Autodesk Inventor part; units mm, degrees
ref_plane "YZ Plane" through (0, 0, 0) normal (1, 0, 0) x (0, 1, 0)
ref_plane "XZ Plane" through (0, 0, 0) normal (0, 1, 0) x (-1, 0, 0)
ref_plane "XY Plane" through (0, 0, 0) normal (0, 0, 1) x (1, 0, 0)
sketch "Sketch1" plane through (0, 0, 0) normal (0, 1, 0) x (-1, 0, 0)
  line L0 (14.0131, 53.7275) -> (-24.0869, 53.7275)
  line L1 (-24.0869, 53.7275) -> (-24.0869, -136.7725)
  line L2 (-24.0869, -136.7725) -> (14.0131, -136.7725)
  line L3 (14.0131, -136.7725) -> (14.0131, 53.7275)
  line L4 (-5.0369, 53.7275) -> (-5.0369, -136.7725)
  point P0 (0, 0)
  dimension "d0" = 38.1
  dimension "d1" = 190.5
revolve "Revolution1" add sketch "Sketch1" angle 360 about axis through (5.0369, 0, 53.7275) along (0, 0, -1) contours L3 L2 L4 L0
sketch "Sketch2" plane through (5.0369, 0, 53.7275) normal (0, 0, 1) x (1, 0, 0)
  circle A0 centre (0, 0) radius 3.175
  point P0 (-5.0369, 0)
  dimension "d3" = 6.35
extrude "Extrusion1" cut sketch "Sketch2" against normal blind 88.9
sketch "Sketch3" plane through (5.0369, 0, -136.7725) normal (0, 0, -1) x (-1, 0, 0)
  circle A0 centre (0, 0) radius 3.175
  circle A1 centre (0, 0) radius 19.05
  circle A2 centre (0, 0) radius 19.05
  line L0 (-16.6914, 9.1815) -> (-16.2946, -9.8685)
  line L1 (-16.2946, -9.8685) -> (-13.1203, -9.8024)
  line L2 (-13.1203, -9.8024) -> (-13.5171, 9.2476)
  line L3 (-13.5171, 9.2476) -> (-16.6914, 9.1815)
  line L4 (0.0496, 19.0499) -> (-0.0211, -19.05)
  line L5 (16.7538, 9.1195) -> (16.2864, -9.9289)
  line L6 (16.2864, -9.9289) -> (13.1124, -9.851)
  line L7 (13.1124, -9.851) -> (13.5798, 9.1974)
  line L8 (13.5798, 9.1974) -> (16.7538, 9.1195)
  point P0 (5.0369, 0)
  dimension "d6" = 3.175
  dimension "d7" = 19.05
extrude "Extrusion2" add sketch "Sketch3" along normal blind 12.7 contours L3 L2 L1 L0 | L8 L5 A1 | A1 L5 L6 L7 L8 | A1 L5 L6
sketch "Sketch4" plane through (21.3316, -9.8685, -136.7725) normal (0.9998, -0.0208, 0) x (0, 0, -1)
  line L0 (12.7, 19.0541) -> (0, 19.0541)
  line L1 (0, 19.0541) -> (0, 0)
  line L2 (0, 0) -> (12.7, 0)
  line L3 (12.7, 0) -> (12.7, 19.0541)
  circle A0 centre (6.35, 9.5271) radius 3.175
  point P0 (-136.7725, 9.4222)
  dimension "d10" = 6.35
extrude "Extrusion3" cut sketch "Sketch4" against normal blind 3149.6 contours A0
sketch "Sketch5" plane through (5.0369, 0, 53.7275) normal (0, 0, 1) x (1, 0, 0)
  circle A0 centre (0, 0) radius 3.175
  circle A1 centre (0, 0) radius 6.35
  point P0 (-5.0369, 0)
  dimension "d13" = 12.7
extrude "Extrusion4" add sketch "Sketch5" along normal blind 12.7
fillet "Fillet1" radius 1.27 4 edges at (-1.3131, 0, 66.4275) (24.0869, 0, 53.7275) (-1.3131, 0, 53.7275) (1.8619, 0, 66.4275)
properties part number "PC3.5-P1"
Input: part model. Units: mm. Frame: model coordinates. A direction names the side the tool comes from. Coordinates: 2 decimals unless noted, no trailing zeros. Order: outer loops, then holes, each group sorted by start corner. A loop starts at its lowest first (then second) coordinate and runs counter-clockwise, first axis right, second up. Notation, with made-up numbers: M 32.5,33.5 L 37.5,33.5 A13 cw 37.5,42.5 Z; hole C 48.25,-4.5 d2. An arc over 180 degrees is marked long. Answer in a Markdown table with one row per item.
(1) Draft query along Y for faces 3 (the flat face through (5, 0, -136.772)), 4 (the cylindrical face through (-1.307, -0.279, 60.006)), 5 (the cylindrical face through (-9.953, -2.789, -142.434)). Return one class per face: pulls with the +Y half, pulls with the -Y half, needs draft (parallel to the pull), parting line crosses it, or undercut.
Numbers:
| item | result |
|---|---|
| face 3 | needs draft |
| face 4 | parting line crosses it |
| face 5 | undercut |
(2) Section query B-B, the plane z = 24.5. Output: boundary loops of the cut face in (x, y) (3 decimals), plus the area to 3 significant figures.
Numbers:
| item | result |
|---|---|
| outline | C 5.037,0 d38.1; hole C 5.037,0 d6.35 |
| area | 1,110 mm^2 |
(3) Section query A-A, the plane z = -96. Output: boundary loops of the cut face in (x, y).
Numbers:
| item | result |
|---|---|
| outline | C 5.04,0 d38.1 |
(4) Material intervals for line 1 (Z direction, x = 15.5, y = -8); line 2 (Y direction, x = 15, z = -74.5); line 3 (Y direction, x = 7.5, z = -94.5), sorted ascending. Write a range as [from, to].
Numbers:
| item | result |
|---|---|
| line 1 | z = [-136.77, 53.73] |
| line 2 | y = [-16.24, 16.24] |
| line 3 | y = [-18.89, 18.89] |
(5) Access query for faces 1 (the cylindrical face through (7.97, 1.22, 14.29)), 2 (the flat face through (20, 0, -149.472)). Directions: +Z, -Z, +X, -X, +Y, -Y. A direction counts if a zero-diameter tool reaches every point of the face in a straight line with its end or side. Return the directions, or none.
Numbers:
| item | result |
|---|---|
| face 1 | +Z |
| face 2 | -Z, +X, -X, +Y, -Y |
(6) Contact query for flat-ended pins moving along their axis: pin 1 Ø6 at (x, y) = (-8, -5.5) entering from +Z; pin 2 Ø16.5 at (x, y) = (2, -7.5) entering from -Z; pin 3 Ø4 at (x, z) = (10, -3) entering from -Y. Output: stop coordinate, or through.
Numbers:
| item | result |
|---|---|
| pin 1 | stops at z = 53.73 |
| pin 2 | stops at z = -136.77 |
| pin 3 | stops at y = -18.82 |
